For this review, take the finished solid that the model builds, in its own axes (mm). A direction names the side the tool comes from. Give positions to 0.01 mm unless a question says otherwise; leave off trailing zeros. Write each loop counter-clockwise with the first axis right and the second up, starting at its lowest first coordinate (ties: lowest second). Pieces come first, ordered by that corner, then holes. Notation, with made-up numbers: (81, -11) -> (120, -11) arc R3 ccw to (120, -7) -> close; hole circle Ø1 at (-25.5, 84). An arc over 180 degrees is marked (long way). Return JSON: item names as keys, results as strings.
from build123d import *

# Parameters (mm, degrees)
F1_DEPTH = 38.1
F2_DEPTH = 19.05


with BuildPart() as f1:
    # F0 (on Front) → F1 (new body, symmetric)
    with BuildSketch(Plane.XZ):
        Polygon((-110.6208127871, 413.4903560323), (-112.7853297752, 408.9222720518), (127, 295.3036472591), (127, 302.2514283657), align=None)
        Polygon((127, -283.5250073743), (-127, -537.5250073743), (-91.0789755157, -573.4460318585), (127, -355.3670563428), align=None)
        with BuildLine():
            Line((-126.9351360354, 379.0599500378), (-127, 378.9230585098))
            ThreePointArc((-127, 378.9230585098), (-12.7, -79.3009744322), (-127, -537.5250073743))
            Line((-127, -537.5250073743), (127, -283.5250073743))
            Line((127, -283.5250073743), (127, 295.3036472591))
            Line((127, 295.3036472591), (-112.7853297752, 408.9222720518))
            Line((-112.7853297752, 408.9222720518), (-126.9351360354, 379.0599500378))
        make_face()
        Polygon((-107.3472207942, 420.3990766491), (-110.6208127871, 413.4903560323), (127, 302.2514283657), (127, 309.5502853394), align=None)
        Polygon((127, 309.5502853394), (127, 316.2741585044), (-105.1827050376, 424.9671580305), (-107.3472207942, 420.3990766491), align=None)
    extrude(amount=F1_DEPTH, both=True)

    # F0 (on Front) → F2 (join, symmetric)
    with BuildSketch(Plane.XZ):
        Polygon((127, -355.3670563428), (-91.0789755157, -573.4460318585), (-46.1776949104, -618.3473124639), (127, -445.1696175535), align=None)
        Polygon((127, 316.2741585044), (127, 379.6250462127), (-80.1566832786, 477.7830840409), (-105.1827050376, 424.9671580305), align=None)
        Polygon((-107.3472207942, 420.3990766491), (-110.6208127871, 413.4903560323), (127, 302.2514283657), (127, 309.5502853394), align=None)
        Polygon((127, 309.5502853394), (127, 316.2741585044), (-105.1827050376, 424.9671580305), (-107.3472207942, 420.3990766491), align=None)
        Polygon((127, 379.6250462127), (127, 386.8607449079), (-77.3567883787, 483.6920952011), (-80.1566832786, 477.7830840409), align=None)
    extrude(amount=F2_DEPTH, both=True)


solid = f1.part
1. The part is to be moulded in two halves that separate along Z. For faces 4 (the flat face through (39.2, 0.27, -532.97)), 5 (the flat face through (12.53, 28.44, 369.86)), 6 (the cylindrical face through (-12.723, -0.533, -72.623)), 7 (the flat face through (9, 19.05, 401)), say which applies: +Z half, -Z half, draft (parallel to the pull), parting line (faces both ways), or undercut.
Results found:
{"face 4": "-Z half", "face 5": "+Z half", "face 6": "undercut", "face 7": "draft"}
2. Add section B-B, the plane x = -26. State the section outline as (y, z) points, plus the area to 3 significant figures.
Results found:
{"outline": "(-38.1, -508.37) -> (-19.05, -508.37) -> (-19.05, -598.17) -> (19.05, -598.17) -> (19.05, -508.37) -> (38.1, -508.37) -> (38.1, -239.85) -> (-38.1, -239.85) -> close; (-38.1, 81.25) -> (38.1, 81.25) -> (38.1, 387.9) -> (19.05, 387.9) -> (19.05, 459.36) -> (-19.05, 459.36) -> (-19.05, 387.9) -> (-38.1, 387.9) -> close", "area": "50,000 mm²"}
3. Add section A-A, the plane y = 1. State the section outline as (x, z) points (3 decimals).
Results found:
{"outline": "(-127, -537.525) -> (-46.178, -618.347) -> (127, -445.17) -> (127, 386.861) -> (-77.357, 483.692) -> (-127, 378.923) arc R975.651 cw to start"}
4. Add section C-C, the plane x = 60. State the section outline as (y, z) points.
Results found:
{"outline": "(-38.1, -422.37) -> (-19.05, -422.37) -> (-19.05, -512.17) -> (19.05, -512.17) -> (19.05, -422.37) -> (38.1, -422.37) -> (38.1, 347.64) -> (19.05, 347.64) -> (19.05, 418.61) -> (-19.05, 418.61) -> (-19.05, 347.64) -> (-38.1, 347.64) -> close"}
5. For pin 1 (8 mm diameter, centred on x = 95, y = 10.5, fed in from +Z); pin 2 (1.5 mm diameter, centred on x = 24, y = -6, fed in from -Z); pin 3 (10 mm diameter, centred on y = -22, z = -451, fed in from -X), all flat-tipped, find the tip position at first contact; note any pin that passes through.
Results found:
{"pin 1": "stops at z = 403.92", "pin 2": "stops at z = -548.92", "pin 3": "stops at x = -88.36"}
6. For faces 1 (the flat face through (16.434, 28.442, -465.933)), 2 (the flat face through (12.53, -28.71, 369.86)), 3 (the flat face through (34, -19.05, -506)), list the 3-axis set-ups (+Z, -Z, +X, -X, +Y, -Y) from which the entire face can be reached by the end or side of a thin tool; tool diameter is ignored.
Results found:
{"face 1": "-Z, +X, +Y", "face 2": "+Z, +X, -Y", "face 3": "-Z, +X, -Y"}
7. Add section D-D, the plane z = 37.5. State the section outline as (x, y) points.
Results found:
{"outline": "(-19.72, -38.1) -> (127, -38.1) -> (127, 38.1) -> (-19.72, 38.1) -> close"}
8. To check wall thickness, follow probe 1 along Y at (x, z) = (-27, 397.5); probe 2 along Z at (x, y) = (-112, 13) (3 decimals); probe 3 along Z at (x, y) = (-98, -4) (3 decimals). State the ranges of each line that lie inside material, in increasing order.
Results found:
{"probe 1": "y = -19.05 to 19.05", "probe 2": "z = -552.525 to -508.141, 349.539 to 410.58", "probe 3": "z = -566.525 to -478.262, 319.66 to 440.126"}
